Source: CAD feature listing. Evaluate the final solid. Frame: model axes, mm. Face numbers are marked on the shaded views. A direction names the side the tool comes from. Give positions to 0.01 mm unless a question says otherwise; leave off trailing zeros. Write each loop counter-clockwise with the first axis right and the second up, starting at its lowest first coordinate (ties: lowest second). Pieces come first, ordered by that corner, then holes. Notation, with made-up numbers: (80.25, 45) -> (113.25, 45) arc R17 cw to (113.25, 62) -> close; hole circle Ø5 at (33, 75). An arc over 180 degrees is marked (long way). Write item = value, one per line.
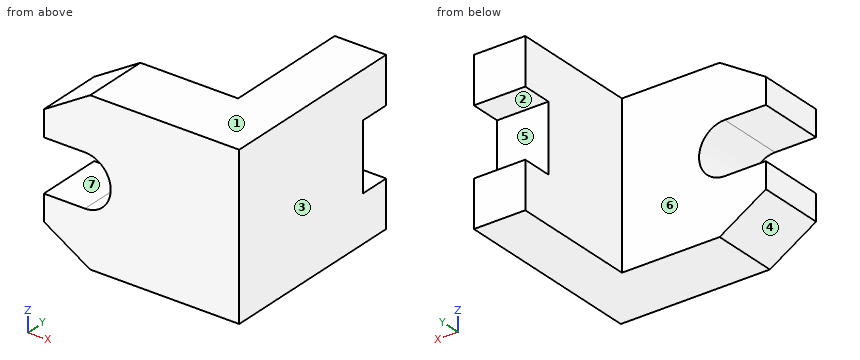
from build123d import *

# Parameters (mm, degrees)
EXTRUDE_1_DEPTH     = 13
SKETCH_2_W          = 10
SKETCH_2_H          = 31
EXTRUDE_2_DEPTH     = 25
SKETCH_3_W          = 10
SKETCH_3_H          = 13
CUT_EXTRUDE_1_DEPTH = 6


with BuildPart() as part:
    # 草图1 → 凸台-拉伸1 (new body)
    with BuildSketch(Plane(origin=(0, 0, 0), x_dir=(1, 0, 0), z_dir=(0, 1, 0))):
        with BuildLine():
            Line((0, 5), (-8, 5))
            Line((-8, 5), (-8, 10))
            Line((-8, 10), (1, 15.5))
            Line((1, 15.5), (30, 15.5))
            Line((30, 15.5), (30, -15.5))
            Line((30, -15.5), (1, -15.5))
            Line((1, -15.5), (-8, -10))
            Line((-8, -10), (-8, -5))
            Line((-8, -5), (0, -5))
            ThreePointArc((0, -5), (5, 0), (0, 5))
        make_face()
    extrude(amount=EXTRUDE_1_DEPTH)

    # 草图2 → 凸台-拉伸2 (add)
    with BuildSketch(Plane(origin=(0, 13, 0), x_dir=(1, 0, 0), z_dir=(0, 1, 0))):
        with Locations((25, 0)):
            Rectangle(SKETCH_2_W, SKETCH_2_H)
    extrude(amount=EXTRUDE_2_DEPTH)

    # 草图3 → 切除-拉伸1 (cut)
    with BuildSketch(Plane(origin=(0, 38, 0), x_dir=(1, 0, 0), z_dir=(0, 1, 0))):
        with Locations((25, 0)):
            Rectangle(SKETCH_3_W, SKETCH_3_H)
    extrude(amount=-CUT_EXTRUDE_1_DEPTH, mode=Mode.SUBTRACT)


solid = part.part
(1) Pull-direction query (Z, two-part tool) for the marked faces 1, 2 and 3; classes: pulls with the +Z half, pulls with the -Z half, needs draft (parallel to the pull), parting line crosses it, or undercut.
Values follow:
face_1 = pulls with the +Z half
face_2 = undercut
face_3 = needs draft
(2) Material intervals for line 1 (X direction, y = 23, z = -1.5); line 2 (Y direction, x = 11, z = 2); line 3 (Y direction, x = 28, z = 0.5), sorted ascending.
Values follow:
line_1 = 20 to 30
line_2 = 0 to 13
line_3 = 0 to 32
(3) First-contact query: pin 1 (12 mm diameter, centred on y = 21, z = 2.5, fed in from -X); pin 2 (4 mm diameter, centred on x = -4.5, y = 8.5, fed in from -Z); pin 3 (6.5 mm diameter, centred on x = -3, y = 7, fed in from +Z). Flat tips, straight axial feed; report the tip coordinate or a pass-through.
Values follow:
pin_1 = 20
pin_2 = -13.36
pin_3 = 15.04
(4) Section query A-A (y = 3.5). Return loops of the section in (x, z).
Values follow:
outline = (-8, -10) -> (1, -15.5) -> (30, -15.5) -> (30, 15.5) -> (1, 15.5) -> (-8, 10) -> (-8, 5) -> (0, 5) arc R5 cw to (0, -5) -> (-8, -5) -> close
(5) Section query B-B (z = 0). Return loops of the section in (x, y), plus the area to 3 significant figures.
Values follow:
outline = (5, 0) -> (30, 0) -> (30, 32) -> (20, 32) -> (20, 13) -> (5, 13) -> close
area = 515 mm2
(6) Section query D-D (z = -8). Return loops of the section in (x, y), plus the area to 3 significant figures.
Values follow:
outline = (-8, 0) -> (30, 0) -> (30, 38) -> (20, 38) -> (20, 13) -> (-8, 13) -> close
area = 744 mm2
(7) Access query for the marked faces 4, 5, 6 and 7. Directions: +Z, -Z, +X, -X, +Y, -Y. A direction counts if a zero-diameter tool reaches every point of the face in a straight line with its end or side. Return the directions, or none.
Values follow:
face_4 = -Z, -X, +Y, -Y
face_5 = +X, -X, +Y
face_6 = +Z, -Z, -X, +Y
face_7 = -X, +Y, -Y
(8) Section query C-C (x = 8). Return loops of the section in (y, z).
Values follow:
outline = (0, -15.5) -> (13, -15.5) -> (13, 15.5) -> (0, 15.5) -> close
